from build123d import *

# Parameters (mm, degrees)
SKETCH2_W           = 176.9
SKETCH2_H           = 176.52
BOSS_EXTRUDE1_DEPTH = 3
SKETCH6_R           = 10
BOSS_EXTRUDE4_DEPTH = 11


with BuildPart() as part:
    # Sketch2 → Boss-Extrude1 (new body)
    with BuildSketch(Plane(origin=(0, 0, 0), x_dir=(1, 0, 0), z_dir=(0, 1, 0))):
        with Locations((88.45, -88.26)):
            Rectangle(SKETCH2_W, SKETCH2_H)
    extrude(amount=BOSS_EXTRUDE1_DEPTH)

    # Sketch6 → Boss-Extrude4 (add)
    with BuildSketch(Plane.XZ):
        with Locations((20, 156.52)):
            Circle(SKETCH6_R)
        with Locations((156.9, 20)):
            Circle(SKETCH6_R)
        with Locations((20, 20)):
            Circle(SKETCH6_R)
        with Locations((156.9, 157.806439708)):
            Circle(SKETCH6_R)
    extrude(amount=BOSS_EXTRUDE4_DEPTH)


solid = part.part
Can you work these out from the model? Positions are in its coordinate system, mm. A direction names the side the tool comes from. Coordinates: 2 decimals unless noted, no trailing zeros. Loops run counter-clockwise (first coordinate to the right, second up) from the corner with the lowest first, then second, coordinate; pieces in that order, holes last. Notation, with made-up numbers: M -36.75,24 L -31.75,24 A18 ccw -31.75,53 Z; hole C -13,54.5 d5. An arc over 180 degrees is marked long. Answer as CSV lines item,"result". Start each with the question number.
1. If I drill on probe 1 along X at (y, z) = (-6.5, 157.5); probe 2 along Y at (x, z) = (14.5, 166.5); probe 3 along Z at (x, y) = (14, -6), over which ranges is the centre line in solid material (lowest first)? Write a range as [from, to].
2. For faces 3 (the face through (25.38, -5.42, 164.95)), 4 (the face through (20, -11, 157)), which set-ups out of +Z, -Z, +X, -X, +Y, -Y let a thin tool reach every point of the face, with its end or its side?
3. Suppose I cut it at D-D, the plane z = 65. List the corners of the cut face in (x, y) for me, plus the area to 3 significant figures.
4. Suppose I cut it at C-C, the plane y = -5.75. List the corners of the cut face in (x, z) for me, plus the area to 3 significant figures.
5. Suppose I cut it at A-A, the plane z = 20. List the corners of the cut face in (x, y) for me, plus the area to 3 significant figures.
6. For pin 1 Ø5 at (x, y) = (139.5, -4.5) entering from -Z; pin 2 Ø1.5 at (x, z) = (124.5, 106.5) entering from -Y, each with a flat end and sliding along its axis, tell me the tip position at first contact or that it passes through.
7. Suppose I cut it at B-B, the plane x = 156.9. List the corners of the cut face in (y, z) for me.
8. Thinking about a two-plate mould opening in Z: for faces 1 (the face through (157, -11, 158)), 2 (the face through (29.54, -5.42, 23)), which applies, +Z half, -Z half, draft (parallel to the pull), parting line (faces both ways), or undercut?
Output:
1,probe 1,"x = [10.05, 29.95], [146.9, 166.9]"
1,probe 2,"y = [0, 3]"
1,probe 3,"z = [12, 28], [148.52, 164.52]"
2,face 3,"-Y"
2,face 4,"+Z, -Z, +X, -X, -Y"
3,outline,"M 0,0 L 176.9,0 L 176.9,3 L 0,3 Z"
3,area,"531 mm^2"
4,outline,"C 20,20 d20; C 20,156.52 d20; C 156.9,20 d20; C 156.9,157.81 d20"
4,area,"1,260 mm^2"
5,outline,"M 0,0 L 10,0 L 10,-11 L 30,-11 L 30,0 L 146.9,0 L 146.9,-11 L 166.9,-11 L 166.9,0 L 176.9,0 L 176.9,3 L 0,3 Z"
5,area,"971 mm^2"
6,pin 1,"passes through"
6,pin 2,"stops at y = 0"
7,outline,"M -11,10 L 0,10 L 0,0 L 3,0 L 3,176.52 L 0,176.52 L 0,167.81 L -11,167.81 L -11,147.81 L 0,147.81 L 0,30 L -11,30 Z"
8,face 1,"draft"
8,face 2,"undercut"
